Could you check a few things on this model? Use its own coordinates, in mm. A direction names the side the tool comes from. Round coordinates to 2 decimals unless told otherwise and drop trailing zeros. Write each loop counter-clockwise with the first axis right and the second up, starting at its lowest first coordinate (ties: lowest second). Pieces come first, ordered by that corner, then holes. Notation, with made-up numbers: (-32, 53.25) -> (-2, 53.25) arc R19 cw to (-2, 58.25) -> close; hole circle Ø8 at (34.25, 62.5). An arc over 180 degrees is marked (long way). Answer in a Markdown table with one row per item.
from build123d import *

# Parameters (mm, degrees)
F2_R     = 4.7625
F3_DEPTH = 7.14475
F5_R     = 1.3208
F6_DEPTH = 14.2875


with BuildPart() as f1:
    # F0 (on Front) → F1 (revolve)
    with BuildSketch(Plane.XZ):
        Polygon((-3.571875, 13.49375), (-3.571875, 0), (3.571875, 0), (3.571875, 13.49375), (0.79375, 13.49375), (0.79375, 14.3002), (-0.79375, 14.3002), (-0.79375, 13.49375), align=None)
    revolve(axis=Axis((0, 0, 0), (1, 0, 0)))

    # F2 (on face) → F3 (cut, through all)
    with BuildSketch(Plane(origin=(-3.571875, 0, 0), x_dir=(0, -1, 0), z_dir=(-1, 0, 0))):
        with Locations((0, 3.96875)):
            Circle(F2_R)
    extrude(amount=-F3_DEPTH, mode=Mode.SUBTRACT)

    # F5 (on offset) → F6 (cut)
    with BuildSketch(Plane.XY.offset(-14.478)):
        Circle(F5_R)
    extrude(amount=F6_DEPTH, mode=Mode.SUBTRACT)


solid = f1.part
1) For faces 4 (the face through (3.572, 0, -3)), 5 (the face through (1.26, 0.4, -7.53)), 6 (the face through (2.16, -4.05, 12.87)), which set-ups out of +Z, -Z, +X, -X, +Y, -Y let a thin tool reach every point of the face, with its end or its side?
Findings:
| item | result |
|---|---|
| face 4 | +Z, -Z, +X, +Y, -Y |
| face 5 | -Z |
| face 6 | +X |
2) Imagine slicing it at A-A, the plane z = 0. Please give me the cut outline in (x, y), plus the area to 3 significant figures.
Findings:
| item | result |
|---|---|
| outline | (-3.57, -13.49) -> (-0.79, -13.49) -> (-0.79, -14.3) -> (0.79, -14.3) -> (0.79, -13.49) -> (3.57, -13.49) -> (3.57, -2.63) -> (-3.57, -2.63) -> close; (-3.57, 2.63) -> (3.57, 2.63) -> (3.57, 13.49) -> (0.79, 13.49) -> (0.79, 14.3) -> (-0.79, 14.3) -> (-0.79, 13.49) -> (-3.57, 13.49) -> close |
| area | 158 mm^2 |
3) Imagine slicing it at D-D, the plane y = 5.75. Please give me the cut outline in (x, z).
Findings:
| item | result |
|---|---|
| outline | (-3.57, -12.21) -> (-0.79, -12.21) -> (-0.79, -13.09) -> (0.79, -13.09) -> (0.79, -12.21) -> (3.57, -12.21) -> (3.57, 12.21) -> (0.79, 12.21) -> (0.79, 13.09) -> (-0.79, 13.09) -> (-0.79, 12.21) -> (-3.57, 12.21) -> close |
4) For pin 1 (2 mm diameter, centred on x = 1.5, y = 10, fed in from +Z); pin 2 (1.5 mm diameter, centred on x = 0, z = 1.5, fed in from +Y); pin 3 (1 mm diameter, centred on x = 0.5, z = 4.5, fed in from -Y), each with a flat end and sliding along its axis, tell me the tip position at first contact or that it passes through.
Findings:
| item | result |
|---|---|
| pin 1 | stops at z = 10.87 |
| pin 2 | stops at y = 14.28 |
| pin 3 | stops at y = -13.73 |
5) Please list where these lines run through material, in increasing order: line 1 (X direction, y = 0, z = -4); line 2 (Z direction, x = -1, y = -2.5); line 3 (Y direction, x = -2.25, z = 8).
Findings:
| item | result |
|---|---|
| line 1 | x = -3.57 to -1.32, 1.32 to 3.57 |
| line 2 | z = -13.26 to -0.08, 8.02 to 13.26 |
| line 3 | y = -10.87 to -2.54, 2.54 to 10.87 |
6) Imagine slicing it at C-C, the plane z = -7. Please give me the cut outline in (x, y).
Findings:
| item | result |
|---|---|
| outline | (-3.57, -11.54) -> (-0.79, -11.54) -> (-0.79, -12.47) -> (0.79, -12.47) -> (0.79, -11.54) -> (3.57, -11.54) -> (3.57, 11.54) -> (0.79, 11.54) -> (0.79, 12.47) -> (-0.79, 12.47) -> (-0.79, 11.54) -> (-3.57, 11.54) -> close; hole circle Ø2.64 at (0, 0) |
7) Thinking about a two-plate mould opening in Z: for faces 1 (the face through (-0.05, -2.56, 7.985)), 2 (the face through (-0.794, -5, 13)), 3 (the face through (-2.2, -4.05, 12.87)), which applies, +Z half, -Z half, draft (parallel to the pull), parting line (faces both ways), or undercut?
Findings:
| item | result |
|---|---|
| face 1 | undercut |
| face 2 | draft |
| face 3 | parting line |
8) Imagine slicing it at B-B, the plane y = -3.25. Please give me the cut outline in (x, z).
Findings:
| item | result |
|---|---|
| outline | (-3.57, -13.1) -> (-0.79, -13.1) -> (-0.79, -13.93) -> (0.79, -13.93) -> (0.79, -13.1) -> (3.57, -13.1) -> (3.57, 0.49) -> (-3.57, 0.49) -> close; (-3.57, 7.45) -> (3.57, 7.45) -> (3.57, 13.1) -> (0.79, 13.1) -> (0.79, 13.93) -> (-0.79, 13.93) -> (-0.79, 13.1) -> (-3.57, 13.1) -> close |
